```python
from build123d import *

# Parameters (mm, degrees)
BOSS_EXTRUDE1_DEPTH = 178.5
CUT_EXTRUDE3_DEPTH  = 169.5
CUT_EXTRUDE2_REACH  = 182.954
SKETCH3_R           = 15.5
CUT_EXTRUDE4_DEPTH  = 2.5
BOSS_EXTRUDE3_DEPTH = 8
BOSS_EXTRUDE4_DEPTH = 133
SKETCH11_R          = 4.35
CUT_EXTRUDE6_DEPTH  = 10
SKETCH12_W          = 6.838099821
SKETCH12_H          = 1.8
CUT_EXTRUDE7_DEPTH  = 133
SKETCH13_W          = 17.8
SKETCH13_H          = 129
BOSS_EXTRUDE5_DEPTH = 4.5
SKETCH16_W          = 16.3
SKETCH16_H          = 129
CUT_EXTRUDE8_DEPTH  = 182.71634489
SKETCH17_R          = 1.6
SKETCH17_W          = 1.75
SKETCH17_H          = 112
CUT_EXTRUDE10_DEPTH = 182.71634489
SKETCH18_R          = 2.9
CUT_EXTRUDE11_DEPTH = 3.2
SKETCH19_R          = 12.5
BOSS_EXTRUDE6_DEPTH = 4
SKETCH20_R          = 4.25
SKETCH20_R_2        = 1.6
CUT_EXTRUDE12_DEPTH = 4
SKETCH21_R          = 2.9
CUT_EXTRUDE13_DEPTH = 2.5
FILLET1_R           = 6
SKETCH22_W          = 5.6
SKETCH22_H          = 8.1
SKETCH22_W_2        = 4.6
SKETCH22_H_2        = 8.3
BOSS_EXTRUDE7_DEPTH = 2.8
BOSS_EXTRUDE8_DEPTH = 2.5


with BuildPart() as part:
    # Sketch1 → Boss-Extrude1 (new body)
    with BuildSketch(Plane.XY):
        Polygon((-21, -0.25), (21, -0.25), (21, -17), (17, -21), (-17, -21), (-21, -17), align=None)
    extrude(amount=BOSS_EXTRUDE1_DEPTH)

    # Sketch4 → Cut-Extrude3 (cut)
    with BuildSketch(Plane.XY.offset(173.5)):
        Polygon((-18.5, -15.964466094), (-15.964466094, -18.5), (15.964466094, -18.5), (18.5, -15.964466094), (18.5, -2.75), (18.5, -0.25), (-18.5, -0.25), (-18.5, -2.75), align=None)
    extrude(amount=-CUT_EXTRUDE3_DEPTH, mode=Mode.SUBTRACT)

    # Sketch3 → Cut-Extrude2 (cut, up to next)
    with BuildSketch(Plane.XY.offset(178.5), mode=Mode.PRIVATE) as cut_extrude2_sk1:
        Circle(SKETCH3_R)
    cut_extrude2_tool1 = extrude(cut_extrude2_sk1.sketch, amount=-CUT_EXTRUDE2_REACH, mode=Mode.PRIVATE) & part.part
    add(cut_extrude2_tool1.solids().sort_by_distance((0, 0, 178.5))[0], mode=Mode.SUBTRACT)

    # Sketch6 → Cut-Extrude4 (cut)
    with BuildSketch(Plane.XY.offset(173.5)):
        with BuildLine():
            Line((-10.974971526, 16.6), (10.974971526, 16.6))
            ThreePointArc((10.974971526, 16.6), (19.9, 0), (10.974971526, -16.6))
            Line((10.974971526, -16.6), (-10.974971526, -16.6))
            ThreePointArc((-10.974971526, -16.6), (-19.9, 0), (-10.974971526, 16.6))
        make_face()
    extrude(amount=-CUT_EXTRUDE4_DEPTH, mode=Mode.SUBTRACT)

    # Sketch7 → Boss-Extrude3 (add)
    with BuildSketch(Plane.XY.offset(171)):
        with BuildLine():
            Line((-6.25, 0), (-6.25, -21))
            Line((-6.25, -21), (6.25, -21))
            Line((6.25, -21), (6.25, 0))
            ThreePointArc((6.25, 0), (0, 6.25), (-6.25, 0))
        make_face()
    extrude(amount=-BOSS_EXTRUDE3_DEPTH)

    # Sketch10 → Boss-Extrude4 (add)
    with BuildSketch(Plane.XY.offset(171)):
        Polygon((-18.5, -1.8), (-18.5, -15.964466094), (-15.964466094, -18.5), (-12.9, -18.5), (-12.9, -1.8), align=None)
    boss_extrude4 = extrude(amount=-BOSS_EXTRUDE4_DEPTH)

    # Mirror1: Boss-Extrude4 across plane
    add(boss_extrude4.mirror(Plane(origin=(0, 0, 0), x_dir=(0, 0, 1), z_dir=(1, 0, 0))))

    # Sketch11 → Cut-Extrude6 (cut)
    with BuildSketch(Plane.XY.offset(171)):
        Circle(SKETCH11_R)
    extrude(amount=-CUT_EXTRUDE6_DEPTH, mode=Mode.SUBTRACT)

    # Sketch12 → Cut-Extrude7 (cut)
    with BuildSketch(Plane(origin=(0, 0, 38), x_dir=(-1, 0, 0), z_dir=(0, 0, -1))):
        with Locations((21.919049911, -0.9)):
            Rectangle(SKETCH12_W, SKETCH12_H)
    extrude(amount=-CUT_EXTRUDE7_DEPTH, mode=Mode.SUBTRACT)

    # Sketch13 → Boss-Extrude5 (add)
    with BuildSketch(Plane(origin=(0, -1.8, 0), x_dir=(1, 0, 0), z_dir=(0, 1, 0))):
        with Locations((-21.8, -104.5)):
            Rectangle(SKETCH13_W, SKETCH13_H)
    extrude(amount=-BOSS_EXTRUDE5_DEPTH)

    # Sketch16 → Cut-Extrude8 (cut, through all)
    with BuildSketch(Plane.XZ.offset(6.3)):
        with Locations((-22.55, 104.5)):
            Rectangle(SKETCH16_W, SKETCH16_H)
    extrude(amount=CUT_EXTRUDE8_DEPTH, mode=Mode.SUBTRACT)

    # Sketch17 → Cut-Extrude10 (cut, through all)
    with BuildSketch(Plane.XZ.offset(6.3)):
        with Locations(Location((-22.55, 164.5, 0), (0, 0, 270))):
            Circle(SKETCH17_R)
        with Locations(Location((-22.55, 44.5, 0), (0, 0, 270))):
            Circle(SKETCH17_R)
        with Locations((-22.55, 104.5)):
            Rectangle(SKETCH17_W, SKETCH17_H)
    extrude(amount=-CUT_EXTRUDE10_DEPTH, mode=Mode.SUBTRACT)

    # Sketch18 → Cut-Extrude11 (cut)
    with BuildSketch(Plane(origin=(0, -1.8, 0), x_dir=(1, 0, 0), z_dir=(0, 1, 0))):
        with Locations(Location((-22.55, -164.5, 0), (0, 0, 270))):
            Circle(SKETCH18_R)
        with Locations(Location((-22.55, -44.5, 0), (0, 0, 270))):
            Circle(SKETCH18_R)
    extrude(amount=-CUT_EXTRUDE11_DEPTH, mode=Mode.SUBTRACT)

    # Sketch19 → Boss-Extrude6 (add)
    with BuildSketch(Plane.XY):
        Circle(SKETCH19_R)
    extrude(amount=BOSS_EXTRUDE6_DEPTH)

    # Sketch20 → Cut-Extrude12 (cut)
    with BuildSketch(Plane.XY):
        Circle(SKETCH20_R)
        with Locations((-8.5, -0.25)):
            Circle(SKETCH20_R_2)
        with Locations(Location((8.5, -0.25, 0), (0, 0, 180))):
            Circle(SKETCH20_R_2)
    extrude(amount=CUT_EXTRUDE12_DEPTH, mode=Mode.SUBTRACT)

    # Sketch21 → Cut-Extrude13 (cut)
    with BuildSketch(Plane.XY.offset(4)):
        with Locations((-8.5, -0.25)):
            Circle(SKETCH21_R)
        with Locations((8.5, -0.25)):
            Circle(SKETCH21_R)
    extrude(amount=-CUT_EXTRUDE13_DEPTH, mode=Mode.SUBTRACT)

    # Fillet1
    fillet1_edges = [part.edges().sort_by_distance(p)[0] for p in [
        (12.49749975, -0.25, 2),
        (-12.49749975, -0.25, 2),
    ]]
    fillet(fillet1_edges, radius=FILLET1_R)

    # Sketch22 → Boss-Extrude7 (add)
    with BuildSketch(Plane(origin=(0, -1.8, 0), x_dir=(1, 0, 0), z_dir=(0, 1, 0))):
        with Locations((15.7, -42.05)):
            Rectangle(SKETCH22_W, SKETCH22_H)
        with Locations((16.2, -166.85)):
            Rectangle(SKETCH22_W_2, SKETCH22_H_2)
    extrude(amount=BOSS_EXTRUDE7_DEPTH)

    # Sketch23 → Boss-Extrude8 (add)
    with BuildSketch(Plane(origin=(0, 0, 173.5), x_dir=(-1, 0, 0), z_dir=(0, 0, -1))):
        with BuildLine():
            Line((-10.974971526, -16.6), (10.974971526, -16.6))
            ThreePointArc((10.974971526, -16.6), (15.448847251, -12.543648537), (18.5, -7.332121112))
            Line((18.5, -7.332121112), (18.5, -15.964466094))
            Line((18.5, -15.964466094), (15.964466094, -18.5))
            Line((15.964466094, -18.5), (-15.964466094, -18.5))
            Line((-15.964466094, -18.5), (-18.5, -15.964466094))
            Line((-18.5, -15.964466094), (-18.5, -7.332121112))
            ThreePointArc((-18.5, -7.332121112), (-15.448847251, -12.543648537), (-10.974971526, -16.6))
        make_face()
    extrude(amount=BOSS_EXTRUDE8_DEPTH)


solid = part.part
```
For this review, take the finished solid that the model builds, in its own axes (mm). A direction names the side the tool comes from. Coordinates: 2 decimals unless noted, no trailing zeros. Order: outer loops, then holes, each group sorted by start corner. A loop starts at its lowest first (then second) coordinate and runs counter-clockwise, first axis right, second up. Notation, with made-up numbers: (-37.5, 47) -> (-33.5, 47) arc R10 cw to (-33.5, 51) -> close; hole circle Ø3 at (-21.5, 69). An arc over 180 degrees is marked (long way). Use CSV: the item, a comma, the result in double quotes. Start each with the question number.
Item 1: We need section C-C, the plane z = 26. Give the boundary of the cut face in (x, y), then the cut area to 3 significant figures.
Item 2: We need section A-A, the plane z = 56.5. Give the boundary of the cut face in (x, y) (3 decimals), then the cut area to 3 significant figures.
Item 3: We need section B-B, the plane x = -2. Give the boundary of the cut face in (y, z).
Item 4: We need section D-D, the plane x = 8.5. Give the boundary of the cut face in (y, z).
Item 5: Insertion check: pin 1 (12 mm diameter, centred on y = -12.5, z = 127.5, fed in from -X); pin 2 (3 mm diameter, centred on x = 16.5, y = 0, fed in from -Z); pin 3 (6.5 mm diameter, centred on x = 9, y = -1.5, fed in from +Z); pin 4 (12 mm diameter, centred on y = 9, z = 120.5, fed in from -X). Each pin has a flat end and moves straight along its axis. Give the tip position at first contact, or say it passes through.
Item 6: For faces 5 (the face through (-23.425, -4, 104)), 6 (the face through (-11.397, -0.122, 2.768)), 7 (the face through (-21, -9, 174)), list the 3-axis set-ups (+Z, -Z, +X, -X, +Y, -Y) from which the entire face can be reached by the end or side of a thin tool; tool diameter is ignored.
Item 7: Wall thickness on probe 1 along X at (y, z) = (-6, 164.5); probe 2 along X at (y, z) = (-12, 140); probe 3 along Z at (x, y) = (3.5, -4.5): over which ranges is each line inside the solid? List them lowest first.
Item 8: Draft analysis for pull direction Z (two halves, no side actions). For faces 1 (the face through (-26, -4, 40)), 2 (the face through (-24, -5, 46)), 3 (the face through (14.019, 0.924, 1.972)), 4 (the face through (0, -17, 178.5)), state which applies: pulls with the +Z half, pulls with the -Z half, needs draft (parallel to the pull), parting line crosses it, or undercut.
Derived:
1,outline,"(-21, -17) -> (-17, -21) -> (17, -21) -> (21, -17) -> (21, -0.25) -> (18.5, -0.25) -> (18.5, -15.96) -> (15.96, -18.5) -> (-15.96, -18.5) -> (-18.5, -15.96) -> (-18.5, -0.25) -> (-21, -0.25) -> close"
1,area,"187 mm^2"
2,outline,"(-30.7, -6.3) -> (-23.425, -6.3) -> (-23.425, -1.8) -> (-30.7, -1.8) -> close; (-21.675, -6.3) -> (-14.4, -6.3) -> (-14.4, -21) -> (17, -21) -> (21, -17) -> (21, -0.25) -> (18.5, -0.25) -> (18.5, -1.8) -> (12.9, -1.8) -> (12.9, -18.5) -> (-12.9, -18.5) -> (-12.9, -1.8) -> (-21.675, -1.8) -> close"
2,area,"310 mm^2"
3,outline,"(-21, 0) -> (-3.75, 0) -> (-3.75, 4) -> (-18.5, 4) -> (-18.5, 163) -> (-3.86, 163) -> (-3.86, 171) -> (-16.6, 171) -> (-16.6, 173.5) -> (-15.37, 173.5) -> (-15.37, 178.5) -> (-21, 178.5) -> close; (3.75, 0) -> (12.34, 0) -> (12.34, 4) -> (3.75, 4) -> close; (3.86, 163) -> (5.92, 163) -> (5.92, 171) -> (3.86, 171) -> close"
4,outline,"(-21, 0) -> (-1.85, 0) -> (-1.85, 1.5) -> (-3.15, 1.5) -> (-3.15, 4) -> (-18.5, 4) -> (-18.5, 171) -> (-16.6, 171) -> (-16.6, 173.5) -> (-12.96, 173.5) -> (-12.96, 178.5) -> (-21, 178.5) -> close; (1.35, 0) -> (9.17, 0) -> (9.17, 4) -> (2.65, 4) -> (2.65, 1.5) -> (1.35, 1.5) -> close"
5,pin 1,"stops at x = -14.4"
5,pin 2,"stops at z = 0"
5,pin 3,"stops at z = 171"
5,pin 4,"passes through"
6,face 5,"+Y, -Y"
6,face 6,"none"
6,face 7,"+Z, -X, +Y, -Y"
7,probe 1,"x = -30.7 to -24.15, -20.95 to -12.9, -6.25 to 6.25, 12.9 to 21"
7,probe 2,"x = -14.4 to -12.9, 12.9 to 21"
7,probe 3,"z = 0 to 4, 163 to 171"
8,face 1,"pulls with the -Z half"
8,face 2,"undercut"
8,face 3,"needs draft"
8,face 4,"pulls with the +Z half"
